Source: CAD feature listing. Evaluate the final solid. Frame: model axes, mm. A direction names the side the tool comes from. Give positions to 0.01 mm unless a question says otherwise; leave off trailing zeros. Loops run counter-clockwise (first coordinate to the right, second up) from the corner with the lowest first, then second, coordinate; pieces in that order, holes last. Notation, with made-up numbers: M 81.25,58 L 139.25,58 A33 cw 139.25,87 Z; hole C 73.25,71.5 d9. An arc over 180 degrees is marked long. Answer in a Markdown table with one row per item.
```python
from build123d import *

# Parameters (mm, degrees)
F0_W      = 1828.8
F0_H      = 609.6
F2_ANGLE  = 90
F2_FACE_W = 1828.8
F2_FACE_H = 609.6
F3_DEPTH  = 367.284
F4_W      = 1854.2
F4_H      = 679.196
F5_DEPTH  = 460.248


with BuildPart() as f2:
    # F0 (on Front) → F2 (revolve)
    with BuildSketch(Plane.XZ):
        Rectangle(F0_W, F0_H)
    revolve(axis=Axis((-199.10112, 0, 609.6), (-1, 0, 0)), revolution_arc=F2_ANGLE)

    # F2_face (on face) → F3 (join)
    with BuildSketch(Plane(origin=(0, 0, 0), x_dir=(-1, 0, 0), z_dir=(0, 1, 0))):
        Rectangle(F2_FACE_W, F2_FACE_H)
    extrude(amount=F3_DEPTH)

    # F4 (on face) → F5 (join)
    with BuildSketch(Plane.XY.offset(609.6)):
        with Locations((0, -609.6)):
            Rectangle(F4_W, F4_H)
    extrude(amount=F5_DEPTH)


solid = f2.part
```
Q1. Section query A-A (x = -448.5). Output: boundary loops of the cut face in (y, z).
Values follow:
| item | result |
|---|---|
| outline | M -949.2,609.6 L -914.4,609.6 A914.4 ccw 0,-304.8 L 367.28,-304.8 L 367.28,304.8 L 0,304.8 A304.8 cw -304.8,609.6 L -270,609.6 L -270,1069.85 L -949.2,1069.85 Z |
Q2. Section query C-C (z = 639). Output: boundary loops of the cut face in (x, y), plus the area to 3 significant figures.
Values follow:
| item | result |
|---|---|
| outline | M -927.1,-949.2 L 927.1,-949.2 L 927.1,-270 L -927.1,-270 Z |
| area | 1,260,000 mm^2 |
Q3. Section query D-D (y = 133.5). Output: boundary loops of the cut face in (x, z), plus the area to 3 significant figures.
Values follow:
| item | result |
|---|---|
| outline | M -914.4,-304.8 L 914.4,-304.8 L 914.4,304.8 L -914.4,304.8 Z |
| area | 1,110,000 mm^2 |
Q4. Mould query, pull axis Z, two halves, no side actions, for faces 1 (the flat face through (-4, -281, 609.6)), 2 (the cylindrical face through (12.802, -213.143, 391.717)), 3 (the flat face through (13, 181, -304.8)), 4 (the flat face through (13, 181, 304.8)). Classes: +Z half, -Z half, draft (parallel to the pull), parting line (faces both ways), or undercut.
Values follow:
| item | result |
|---|---|
| face 1 | undercut |
| face 2 | undercut |
| face 3 | -Z half |
| face 4 | +Z half |
Q5. Ray query, probe 1 along Y at (x, z) = (429.5, 968); probe 2 along X at (y, z) = (-546.5, 59.5); probe 3 along Z at (x, y) = (-394, 310.5). Return the intervals inside material, ascending. Write a range as from..to.
Values follow:
| item | result |
|---|---|
| probe 1 | -949.2..-270 |
| probe 2 | -914.4..914.4 |
| probe 3 | -304.8..304.8 |
Q6. Section query B-B (y = -425). Output: boundary loops of the cut face in (x, z), plus the area to 3 significant figures.
Values follow:
| item | result |
|---|---|
| outline | M -927.1,609.6 L -914.4,609.6 L -914.4,-200.03 L 914.4,-200.03 L 914.4,609.6 L 927.1,609.6 L 927.1,1069.85 L -927.1,1069.85 Z |
| area | 2,330,000 mm^2 |
Q7. Reachability of faces 5 (the flat face through (-13, -270.002, 837)), 6 (the flat face through (-914.4, -283, 146)), 7 (the flat face through (-13, -949.198, 837)), 8 (the flat face through (-13, -605, 1069.848)), 9 (the flat face through (914.4, -283, 146)) from +Z, -Z, +X, -X, +Y, -Y: full face, straight path, thin tool, end or side. Return the list, or none.
Values follow:
| item | result |
|---|---|
| face 5 | +Z, +X, -X, +Y |
| face 6 | -Z, -X, +Y, -Y |
| face 7 | +Z, -Z, +X, -X, -Y |
| face 8 | +Z, +X, -X, +Y, -Y |
| face 9 | -Z, +X, +Y, -Y |
Q8. Contact query for flat-ended pins moving along their axis: pin 1 Ø5 at (x, z) = (-215.5, 893) entering from +Y; pin 2 Ø2 at (x, y) = (-710.5, -43.5) entering from +Z; pin 3 Ø8 at (y, z) = (-277, 304.5) entering from +X. Output: stop coordinate, or through.
Values follow:
| item | result |
|---|---|
| pin 1 | y = -270 |
| pin 2 | z = 308.07 |
| pin 3 | x = 914.4 |
